Autodesk Inventor part; units mm, degrees
ref_plane "YZ Plane" through (0, 0, 0) normal (1, 0, 0) x (0, 1, 0)
ref_plane "XZ Plane" through (0, 0, 0) normal (0, 1, 0) x (-1, 0, 0)
ref_plane "XY Plane" through (0, 0, 0) normal (0, 0, 1) x (1, 0, 0)
sketch "スケッチ2" plane through (0, 0, 0) normal (0, 0, 1) x (1, 0, 0)
  line L0 (0, -49.4975) -> (49.4975, 0)
  line L1 (49.4975, 0) -> (0, 49.4975)
  line L2 (0, 49.4975) -> (-49.4975, 0)
  line L3 (-49.4975, 0) -> (0, -49.4975)
  line L4 (0, -49.4975) -> (0, 49.4975) construction
  line L5 (49.4975, 0) -> (-49.4975, 0) construction
  circle A0 centre (-5, 35) radius 1.75
  circle A1 centre (5, 35) radius 1.75
  circle A2 centre (-35, -5) radius 1.75
  circle A3 centre (-35, 5) radius 1.75
  circle A4 centre (5, -35) radius 1.75
  circle A5 centre (-5, -35) radius 1.75
  circle A6 centre (35, 5) radius 1.75
  circle A7 centre (35, -5) radius 1.75
  line L6 (-24.7487, 24.7487) -> (24.7487, -24.7487) construction
  line L7 (24.7487, 24.7487) -> (-24.7487, -24.7487) construction
  circle A8 centre (17.6777, 17.6777) radius 2.75
  circle A9 centre (-17.6777, 17.6777) radius 1.75
  circle A10 centre (-17.6777, -17.6777) radius 2.75
  circle A11 centre (17.6777, -17.6777) radius 1.75
  circle A12 centre (-30, 0) radius 1.75
  circle A13 centre (-40, 0) radius 1.75
  line L8 (-35, -5) -> (-35, 5) construction
  circle A14 centre (0, -30) radius 1.75
  circle A15 centre (0, -40) radius 1.75
  circle A16 centre (30, 0) radius 1.75
  circle A17 centre (40, 0) radius 1.75
  circle A18 centre (0, 30) radius 1.75
  circle A19 centre (0, 40) radius 1.75
  point P0 (0, 0)
  dimension "d1" = 3.5
  dimension "d2" = 5
  dimension "d3" = 35
  dimension "d6" = 360
  dimension "d12" = 5.5
  dimension "d13" = 3.5
  dimension "d14" = 25
  dimension "d15" = 25
  dimension "d29" = 70
  dimension "d30" = 5
  dimension "d31" = 5
  dimension "d34" = 360
extrude "押し出し1" add sketch "スケッチ2" along normal blind 4
chamfer "面取り1" distance 5 angle 45 4 edges at (0, -49.4975, 2) (49.4975, 0, 2) (0, 49.4975, 2) (-49.4975, 0, 2)
properties part number "_3D プリント"
Geometry: final body of the model. Coordinates: model frame, mm. Round coordinates to 2 decimals unless told otherwise and drop trailing zeros. Order: outer loops, then holes, each group sorted by start corner. A loop starts at its lowest first (then second) coordinate and runs counter-clockwise, first axis right, second up. Notation, with made-up numbers: M -39.75,12 L 0.25,12 A17 cw 0.25,32 Z; hole C -16,-20 d1. An arc over 180 degrees is marked long. Use one line per item in the form item = value. Start each with the question number.
Q1. Cut plane D-D (x = 40). Return loops of the section in (y, z), and give its area (3 significant figures).
Q2. Cut plane B-B (z = 2.55). Count the separate pieces of the cut face and the enclosed holes in it, and give its area (3 significant figures).
Q3. Material intervals for line 1 (Y direction, x = 0, z = 2.55); line 2 (Y direction, x = 5, z = 0.75); line 3 (Y direction, x = 19, z = 0.5), sorted ascending. Write a range as [from, to].
Q4. Cut plane C-C (x = 5). Return loops of the section in (y, z).
Q5. Mould query, pull axis Y, two halves, no side actions, for faces 1 (the face through (-25, -24.5, 2)), 2 (the face through (-0.38, -38.29, 1.97)), 3 (the face through (25, 24.5, 2)). Classes: +Y half, -Y half, draft (parallel to the pull), parting line (faces both ways), or undercut.
Q6. Cut plane A-A (y = 0). Return loops of the section in (x, z).
Q7. Pin query (flat end, axial travel): pin 1 Ø1 at (y, z) = (-18.5, 0.5) entering from +X; pin 2 Ø1.5 at (x, z) = (6, 3) entering from +Y. Return the tip coordinate at first contact, or that it passes through.
Geometry results:
q1.outline = M -9.5,0 L -1.75,0 L -1.75,4 L -9.5,4 Z; M 1.75,0 L 9.5,0 L 9.5,4 L 1.75,4 Z
q1.area = 62.0 mm^2
q2.separate_pieces = 1
q2.enclosed_holes = 20
q2.area = 4,630 mm^2
q3.line_1 = [-45.96, -41.75], [-38.25, -31.75], [-28.25, 28.25], [31.75, 38.25], [41.75, 45.96]
q3.line_2 = [-44.5, -36.75], [-33.25, 33.25], [36.75, 44.5]
q3.line_3 = [-30.5, -18.82], [-16.53, 15.27], [20.09, 30.5]
q4.outline = M -44.5,0 L -36.75,0 L -36.75,4 L -44.5,4 Z; M -33.25,0 L 33.25,0 L 33.25,4 L -33.25,4 Z; M 36.75,0 L 44.5,0 L 44.5,4 L 36.75,4 Z
q5.face_1 = -Y half
q5.face_2 = undercut
q5.face_3 = +Y half
q6.outline = M -45.96,0 L -41.75,0 L -41.75,4 L -45.96,4 Z; M -38.25,0 L -31.75,0 L -31.75,4 L -38.25,4 Z; M -28.25,0 L 28.25,0 L 28.25,4 L -28.25,4 Z; M 31.75,0 L 38.25,0 L 38.25,4 L 31.75,4 Z; M 41.75,0 L 45.96,0 L 45.96,4 L 41.75,4 Z
q7.pin_1 = 31.5
q7.pin_2 = 44.25
